Part model, mm, in its own coordinate system. Give positions to 0.01 mm unless a question says otherwise; leave off trailing zeros. Order: outer loops, then holes, each group sorted by start corner. A loop starts at its lowest first (then second) coordinate and runs counter-clockwise, first axis right, second up. Notation, with made-up numbers: (-26.75, 5) - (-17.75, 5) arc R19 cw to (-17.75, 42) - close; hole circle Ø9 at (57, 63.25). An arc over 180 degrees is marked (long way). One line per item, written item: value.
```python
from build123d import *

# Parameters (mm, degrees)
BOSS_EXTRU_2_DEPTH      = 10
ENL_V_MAT_EXTRU_1_DEPTH = 10


with BuildPart() as part:
    # Esquisse1 → Boss.-Extru.2 (new body)
    with BuildSketch(Plane.XY):
        Polygon((0, 0), (390, 0), (390, 90), (380, 90), (380, 190), (390, 190), (390, 280), (0, 280), (0, 190), (10, 190), (10, 90), (0, 90), align=None)
    extrude(amount=BOSS_EXTRU_2_DEPTH)

    # Esquisse3 → Enlèv. mat.-Extru.1 (cut)
    with BuildSketch(Plane.XY.offset(10)):
        Polygon((70, 100), (110, 60), (280, 60), (320, 100), (320, 200), (300, 220), (90, 220), (70, 200), align=None)
    extrude(amount=-ENL_V_MAT_EXTRU_1_DEPTH, mode=Mode.SUBTRACT)


solid = part.part
```
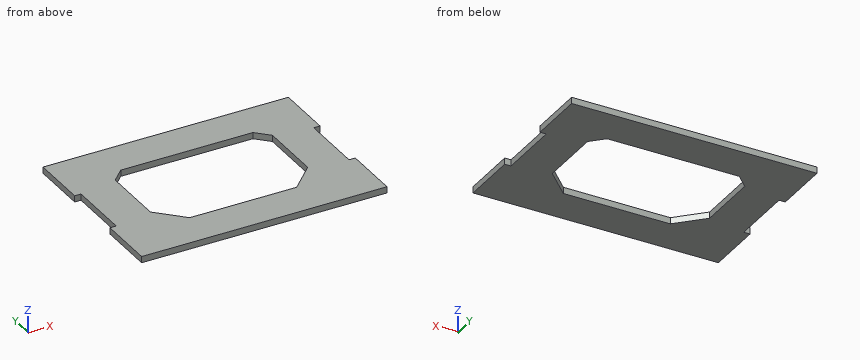
1) Drop flat-ended pins along their axis: P1, Ø1, axis at x = 234.5, y = 249.5, coming from the -Z side; P2, Ø3, axis at y = 137.5, z = 6.5, coming from the -X side; P3, Ø5, axis at y = 138.5, z = 4, coming from the +X side. Give the stop position or say it passes through.
Answer:
P1: stops at z = 0
P2: stops at x = 10
P3: stops at x = 380
2) Wall check: line 1 along Y through (x, z) = (132, 7.5); line 2 along X through (y, z) = (132.5, 4.25); line 3 along Y through (x, z) = (285, 5.25). Give the ranges that are in metal, low to high. Write a range as [from, to].
Answer:
line 1: y = [0, 60], [220, 280]
line 2: x = [10, 70], [320, 380]
line 3: y = [0, 65], [220, 280]
3) Slice it at A-A on y = 128.5. Write the cut outline in (x, z), then the cut area to 3 significant figures.
Answer:
outline: (10, 0) - (70, 0) - (70, 10) - (10, 10) - close; (320, 0) - (380, 0) - (380, 10) - (320, 10) - close
area: 1,200 mm2
4) Slice it at B-B on x = 76. Write the cut outline in (y, z), then the cut area to 3 significant figures.
Answer:
outline: (0, 0) - (94, 0) - (94, 10) - (0, 10) - close; (206, 0) - (280, 0) - (280, 10) - (206, 10) - close
area: 1,680 mm2
5) Slice it at C-C on z = 6.5. Write the cut outline in (x, y), then the cut area to 3 significant figures.
Answer:
outline: (0, 0) - (390, 0) - (390, 90) - (380, 90) - (380, 190) - (390, 190) - (390, 280) - (0, 280) - (0, 190) - (10, 190) - (10, 90) - (0, 90) - close; hole (70, 100) - (110, 60) - (280, 60) - (320, 100) - (320, 200) - (300, 220) - (90, 220) - (70, 200) - close
area: 69,200 mm2
